Build history of the part. All positions in model axes, mm. A direction names the side the tool comes from. Coordinates: 2 decimals unless noted, no trailing zeros. Order: outer loops, then holes, each group sorted by start corner. A loop starts at its lowest first (then second) coordinate and runs counter-clockwise, first axis right, second up. Notation, with made-up numbers: (-10.75, 44) - (38.25, 44) arc R27 ccw to (38.25, 80) - close; hole circle Ø4 at (67, 84). An arc over 180 degrees is marked (long way). One line per item, written item: value.
from build123d import *

# Parameters (mm, degrees)
PAD004_DEPTH    = 8.2
SKETCH014_W     = 28.5
SKETCH014_H     = 6.1
PAD005_DEPTH    = 1.8
SKETCH015_R     = 2.9
POCKET004_DEPTH = 0.6
SKETCH016_W     = 2.05
SKETCH016_H     = 6.1
POCKET005_DEPTH = 1.8
SKETCH018_R     = 1.05
POCKET007_DEPTH = 6
POCKET006_DEPTH = 4
SKETCH019_R     = 2.55
POCKET008_DEPTH = 7.5
SKETCH020_R     = 7
POCKET_DEPTH    = 3


with BuildPart() as stage_1_railguide:
    # Sketch013 → Pad004 (new body)
    with BuildSketch(Plane.XY):
        with BuildLine():
            Line((0, 0), (28.5, 0))
            Line((28.5, 0), (28.5, 22.75))
            Line((28.5, 22.75), (14, 22.75))
            Line((14, 22.75), (14, 22.5))
            ThreePointArc((11, 19.5), (13.12132, 20.37868), (14, 22.5))
            Line((11, 19.5), (0, 19.5))
            Line((0, 19.5), (0, 0))
        make_face()
    extrude(amount=PAD004_DEPTH)

    # Sketch014 (on Face9 of Pad004) → Pad005 (join)
    with BuildSketch(Plane.XY.offset(8.2)):
        with Locations((14.25, 9.75)):
            Rectangle(SKETCH014_W, SKETCH014_H)
    extrude(amount=PAD005_DEPTH)

    # Sketch015 (on Face11 of Pad005) → Pocket004 (cut)
    with BuildSketch(Plane.XY.offset(10)):
        with Locations((8.735056, 9.75)):
            Circle(SKETCH015_R)
    extrude(amount=-POCKET004_DEPTH, mode=Mode.SUBTRACT)

    # Sketch016 (on Face10 of Pocket004) → Pocket005 (cut)
    with BuildSketch(Plane.XY.offset(10)):
        with Locations((15.5, 9.75)):
            Rectangle(SKETCH016_W, SKETCH016_H)
        Polygon((21.525, 12.8), (21.525, 6.7), (19.475, 6.7), (19.475, 12.8), (20.5, 12.8), align=None)
        with Locations((25.5, 9.75)):
            Rectangle(SKETCH016_W, SKETCH016_H)
    extrude(amount=-POCKET005_DEPTH, mode=Mode.SUBTRACT)


with BuildPart() as body:
    # Body006 base: copy of Stage#1(RailGuide)
    add(stage_1_railguide.part)

    # Sketch018 (on Face19 of Clone001) → Pocket007 (cut)
    with BuildSketch(Plane.XY.offset(8.2)):
        with BuildLine():
            Line((14, 22.75), (26.9, 22.75))
            Line((26.9, 22.75), (26.9, 16.25))
            Line((26.355184, 16.25), (26.9, 16.25))
            ThreePointArc((21.044816, 16.25), (23.7, 14.75), (26.355184, 16.25))
            Line((20.45, 16.25), (21.044816, 16.25))
            Line((19.855184, 16.25), (20.45, 16.25))
            ThreePointArc((14.544816, 16.25), (17.2, 14.75), (19.855184, 16.25))
            Line((14, 16.25), (14.544816, 16.25))
            Line((14, 16.25), (14, 22.75))
        make_face()
        with Locations((17.2, 17.85)):
            Circle(SKETCH018_R, mode=Mode.SUBTRACT)
        with Locations((23.7, 17.85)):
            Circle(SKETCH018_R, mode=Mode.SUBTRACT)
    extrude(amount=-POCKET007_DEPTH, mode=Mode.SUBTRACT)


with BuildPart() as body008:
    # Body005 base: copy of Stage#1(RailGuide)
    add(stage_1_railguide.part)

    # Sketch017 (on Face19 of Clone) → Pocket006 (cut)
    with BuildSketch(Plane.XY.offset(8.2)):
        with BuildLine():
            Line((0, 5.7), (13.475, 5.7))
            ThreePointArc((13.475, 5.7), (14.182107, 5.992893), (14.475, 6.7))
            Line((14.475, 6.7), (14.475, 16.75))
            Line((14.475, 16.75), (16.525, 16.75))
            Line((16.525, 16.75), (16.525, 5.7))
            Line((16.525, 5.7), (18.475, 5.7))
            ThreePointArc((18.475, 5.7), (19.182107, 5.992893), (19.475, 6.7))
            Line((19.475, 6.7), (19.475, 16.75))
            Line((19.475, 16.75), (21.525, 16.75))
            Line((21.525, 16.75), (21.525, 5.699968))
            Line((21.525, 5.699968), (23.475, 5.699968))
            ThreePointArc((23.475, 5.699968), (24.182107, 5.992862), (24.475, 6.699968))
            Line((24.475, 6.699968), (24.475, 16.75))
            Line((24.475, 16.75), (26.525, 16.75))
            Line((26.525, 16.75), (26.525, 5.7))
            ThreePointArc((24.475, 3.65), (25.924569, 4.250431), (26.525, 5.7))
            Line((24.475, 3.65), (0, 3.65))
            Line((0, 3.65), (0, 5.7))
        make_face()
    extrude(amount=-POCKET006_DEPTH, mode=Mode.SUBTRACT)

    # Sketch019 (on Face37 of Pocket006) → Pocket008 (cut)
    with BuildSketch(Plane.XY.offset(9.4)):
        with Locations((8.735056, 9.75)):
            Circle(SKETCH019_R)
    extrude(amount=-POCKET008_DEPTH, mode=Mode.SUBTRACT)

    # Sketch020 (on Face4 of Pocket008) → Pocket (cut)
    with BuildSketch(Plane(origin=(0, 0, 0), x_dir=(1, 0, 0), z_dir=(0, 0, -1))):
        with Locations((8.735056, -9.75)):
            Circle(SKETCH020_R)
    extrude(amount=-POCKET_DEPTH, mode=Mode.SUBTRACT)

    # Common: intersect Body
    add(body.part, mode=Mode.INTERSECT)


solid = body008.part
1. Probe line 1 along Y through (x, z) = (2.5, 5.5); line 2 along X through (y, z) = (9.75, 1.85); line 3 along X through (y, z) = (16.5, 5.25). List the from-to ranges inside material, lowest first.
Values found:
line 1: y = 0 to 3.65, 5.7 to 19.5
line 2: x = 0 to 1.74, 15.74 to 28.5
line 3: x = 0 to 14, 26.9 to 28.5
2. Flat gauge pins, fed straight in: P1, Ø6, axis at x = 9.5, y = 10, coming from the -Z side; P2, Ø0.9, axis at x = 23, z = 9, coming from the -Y side; P3, Ø0.6, axis at x = 26.5, z = 4.5, coming from the +Y side. Where does each tip first touch, or does it go through?
Values found:
P1: stops at z = 3
P2: stops at y = 6.7
P3: stops at y = 16.25
3. 3-axis set-ups, long thin cutter, end or side, ignore diameter. For faces 4 (the face through (17, 18, 8.2)), 5 (the face through (24.174, 5.985, 6.228)), 6 (the face through (27, 6.7, 9)), 7 (the face through (12, 3.65, 6)): which of +Z, -Z, +X, -X, +Y, -Y reach the whole face in a straight line?
Values found:
face 4: +Z, +X, -X, +Y
face 5: +Z
face 6: +Z, +X, -X, -Y
face 7: +Z, -X
4. Band-saw the part on C-C, the plane x = 9.5. Give the cut face in (y, z).
Values found:
outline: (0, 0) - (2.79, 0) - (2.79, 3) - (7.32, 3) - (7.32, 9.4) - (6.95, 9.4) - (6.95, 10) - (6.7, 10) - (6.7, 8.2) - (5.7, 8.2) - (5.7, 4.2) - (3.65, 4.2) - (3.65, 8.2) - (0, 8.2) - close; (12.18, 3) - (16.71, 3) - (16.71, 0) - (19.5, 0) - (19.5, 8.2) - (12.8, 8.2) - (12.8, 10) - (12.55, 10) - (12.55, 9.4) - (12.18, 9.4) - close
5. Band-saw the part on B-B, the plane y = 9.75. Give the cut face in (x, z) (3 decimals), and give its area (3 significant figures).
Values found:
outline: (0, 0) - (1.735, 0) - (1.735, 3) - (6.185, 3) - (6.185, 9.4) - (5.835, 9.4) - (5.835, 10) - (0, 10) - close; (11.285, 3) - (15.735, 3) - (15.735, 0) - (28.5, 0) - (28.5, 10) - (26.525, 10) - (26.525, 4.2) - (24.475, 4.2) - (24.475, 10) - (21.525, 10) - (21.525, 4.2) - (19.475, 4.2) - (19.475, 10) - (16.525, 10) - (16.525, 4.2) - (14.475, 4.2) - (14.475, 10) - (11.635, 10) - (11.635, 9.4) - (11.285, 9.4) - close
area: 171 mm2
6. Two-plate mould, pull along Y, no slides. Class faces 1 (the face through (14.174, 5.985, 6.228)), 2 (the face through (23, 22.75, 2)), 3 (the face through (14, 19, 5)): pulls with the +Y half, pulls with the -Y half, needs draft (parallel to the pull), parting line crosses it, or undercut.
Values found:
face 1: undercut
face 2: pulls with the +Y half
face 3: needs draft
7. Band-saw the part on A-A, the plane z = 9. Give the cut face in (x, y) (3 decimals), and give its area (3 significant figures).
Values found:
outline: (0, 6.7) - (14.475, 6.7) - (14.475, 12.8) - (0, 12.8) - close; (16.525, 6.7) - (19.475, 6.7) - (19.475, 12.8) - (16.525, 12.8) - close; (21.525, 6.7) - (24.475, 6.7) - (24.475, 12.8) - (21.525, 12.8) - close; (26.525, 6.7) - (28.5, 6.7) - (28.5, 12.8) - (26.525, 12.8) - close; hole circle Ø5.1 at (8.735, 9.75)
area: 116 mm2
8. Band-saw the part on D-D, the plane z = 1.25. Give the cut face in (x, y).
Values found:
outline: (0, 0) - (28.5, 0) - (28.5, 22.75) - (14, 22.75) - (14, 22.5) arc R3 cw to (11, 19.5) - (0, 19.5) - close; hole circle Ø14 at (8.74, 9.75)
